Geometry check sheet. Reference: the model listing, model coordinates, mm. Give positions to 0.01 mm unless a question says otherwise; leave off trailing zeros. Write each loop counter-clockwise with the first axis right and the second up, starting at its lowest first coordinate (ties: lowest second). Pieces come first, ordered by that corner, then holes.
(1) Depth check by flat-ended pin: P1, Ø3.5, axis at y = 0, z = -108.5, coming from the -X side. Enter the tip coordinate at first touch or a pass-through.
(2) Cross-section at A-A (x = -0.75). Count the separate pieces of the cut face and the enclosed holes in it, and give its area (3 significant figures).
(3) Thickness scan on line 1 along Z through (x, y) = (0.5, 0); line 2 along Y through (x, z) = (0.4, -108.5); line 3 along Z through (x, y) = (-0.55, -5). Record the ranges inside material, lowest first.
(4) Cross-section at B-B (y = -17). Record the boundary of the cut face in (x, z), and give its area (3 significant figures).
```python
from build123d import *

# Parameters (mm, degrees)
F1_W     = 50
F1_H     = 277
F1_R     = 1.5875
F2_DEPTH = 1.5875
F3_R     = 24.99999


# Not quite as in the source:
# - a fillet or chamfer is up to 0.001 mm smaller than in the source, because OpenCascade refuses the exact size
# - a length typed as a fraction of an inch, garbled in the dataset ("3 / 203.2 mm" for 3/8 in), is restored


with BuildPart() as f2:
    # F1 (on Right) → F2 (new body, symmetric)
    with BuildSketch(Plane.YZ):
        Rectangle(F1_W, F1_H)
        with Locations((0, -108.5)):
            Circle(F1_R, mode=Mode.SUBTRACT)
        with Locations((0, 108.5)):
            Circle(F1_R, mode=Mode.SUBTRACT)
    extrude(amount=F2_DEPTH, both=True)

    # F3 (radius 25 in the source; OpenCascade refuses exactly that, so slightly less here)
    f3_edges = [f2.edges().sort_by_distance(p)[0] for p in [
        (0, -25, 138.5),
        (0, 25, 138.5),
    ]]
    fillet(f3_edges, radius=F3_R)


solid = f2.part
```
Reply:
1. P1: stops at x = -1.59
2. separate pieces: 1
2. enclosed holes: 2
2. area: 13,600 mm2
3. line 1: z = -138.5 to -110.09, -106.91 to 106.91, 110.09 to 138.5
3. line 2: y = -25 to -1.59, 1.59 to 25
3. line 3: z = -138.5 to 137.99
4. outline: (-1.59, -138.5) - (1.59, -138.5) - (1.59, 131.83) - (-1.59, 131.83) - close
4. area: 858 mm2
